Verification items for the finished model (mm, model axes). Round coordinates to 2 decimals unless told otherwise and drop trailing zeros. Order: outer loops, then holes, each group sorted by start corner. A loop starts at its lowest first (then second) coordinate and runs counter-clockwise, first axis right, second up. Notation, with made-up numbers: M 39.25,42.25 L 80.25,42.25 A14 ccw 80.25,48.25 Z; hole C 61.25,32.25 d2. An arc over 180 degrees is marked long. Return JSON: item names as keys, results as strings. Group by question number.
from build123d import *

# Parameters (mm, degrees)
SKETCH1_R                  = 0.5
BOSS_EXTRUDE1_DEPTH        = 4.5
SKETCH2_R                  = 0.75
BOSS_EXTRUDE2_DEPTH        = 0.1
DOME1_FACE_RADIUS          = 0.75
DOME1_HEIGHT               = 0.25
FILLET1_R                  = 0.05
MIRROR2_COPY_1_FACE_RADIUS = 0.75
MIRROR2_COPY_1_HEIGHT      = 0.25
FILLET1_OF_MIRROR2_R       = 0.05


with BuildPart() as part:
    # Sketch1 → Boss-Extrude1 (new, symmetric)
    with BuildSketch(Plane.XY):
        Circle(SKETCH1_R)
    extrude(amount=BOSS_EXTRUDE1_DEPTH, both=True)

    # Sketch2 → Boss-Extrude2 (add)
    with BuildSketch(Plane.XY.offset(4.5)):
        Circle(SKETCH2_R)
    boss_extrude2 = extrude(amount=BOSS_EXTRUDE2_DEPTH)

    # Dome1: an elliptical dome of height H over a round flat face of radius A is half a spheroid: the quarter ellipse of half axes A and H revolved about the face's axis
    with BuildSketch(Plane((0, 0, 4.6), x_dir=(0, 1, 0), z_dir=(1, 0, 0)), mode=Mode.PRIVATE) as dome1_quarter:
        Ellipse(DOME1_FACE_RADIUS, DOME1_HEIGHT)
        Rectangle(DOME1_FACE_RADIUS, DOME1_HEIGHT, align=(Align.MIN, Align.MIN), mode=Mode.INTERSECT)
    revolve(dome1_quarter.sketch, axis=Axis((0, 0, 4.6), (0, 0, 1)))

    # Fillet1
    fillet1_edges = [part.edges().sort_by_distance(p)[0] for p in [
        (-0.75, 0, 4.5),
    ]]
    fillet(fillet1_edges, radius=FILLET1_R)

    # Mirror2: Boss-Extrude2 across plane
    add(boss_extrude2.mirror(Plane.XY))

    # Mirror2 copy 1: an elliptical dome of height H over a round flat face of radius A is half a spheroid: the quarter ellipse of half axes A and H revolved about the face's axis
    with BuildSketch(Plane((0, 0, -4.6), x_dir=(0, -1, 0), z_dir=(1, 0, 0)), mode=Mode.PRIVATE) as mirror2_copy_1_quarter:
        Ellipse(MIRROR2_COPY_1_FACE_RADIUS, MIRROR2_COPY_1_HEIGHT)
        Rectangle(MIRROR2_COPY_1_FACE_RADIUS, MIRROR2_COPY_1_HEIGHT, align=(Align.MIN, Align.MIN), mode=Mode.INTERSECT)
    revolve(mirror2_copy_1_quarter.sketch, axis=Axis((0, 0, -4.6), (0, 0, -1)))

    # Fillet1 of Mirror2
    fillet1_of_mirror2_edges = [part.edges().sort_by_distance(p)[0] for p in [
        (-0.75, 0, -4.5),
    ]]
    fillet(fillet1_of_mirror2_edges, radius=FILLET1_OF_MIRROR2_R)


solid = part.part
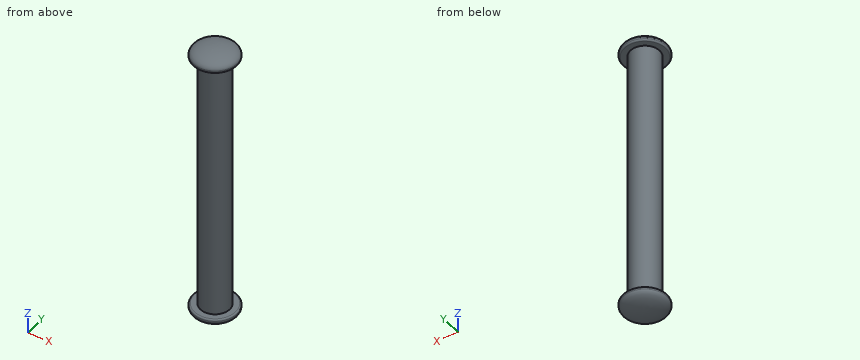
1. Cross-section at A-A (z = -3.75). Enter the section's corners in (x, y), plus the area to 3 significant figures.
2. Go/stop test with a flat-tipped pin: pin 1 (0.7 mm diameter, centred on x = -0.5, y = 0.5, fed in from +Z). Record where the tip stops, or that it passes through.
3. Thickness scan on line 1 along Y through (x, z) = (-0.05, -2.25); line 2 along X through (y, z) = (-0.2, -4); line 3 along Z through (x, y) = (-0.25, -0.4). Record the ranges inside material, lowest first. Write a range as from..to.
Computed:
{
 "1": {"outline": "C 0,0 d1", "area": "0.785 mm²"},
 "2": {"pin 1": "stops at z = 4.82"},
 "3": {"line 1": "y = -0.5..0.5", "line 2": "x = -0.46..0.46", "line 3": "z = -4.79..4.79"}
}
